Here's how the part is built. I have some questions about the finished solid (model axes, mm). Round coordinates to 2 decimals unless told otherwise and drop trailing zeros. Order: outer loops, then holes, each group sorted by start corner. A loop starts at its lowest first (then second) coordinate and runs counter-clockwise, first axis right, second up. Notation, with made-up numbers: (30.25, 79) -> (37.25, 79) arc R23 ccw to (37.25, 95) -> close; hole circle Ø4 at (26, 75.5). An arc over 180 degrees is marked (long way). Answer in a Markdown table with one row per item.
Autodesk Inventor part; units mm, degrees
ref_plane "YZ Plane" through (0, 0, 0) normal (1, 0, 0) x (0, 1, 0)
ref_plane "XZ Plane" through (0, 0, 0) normal (0, 1, 0) x (-1, 0, 0)
ref_plane "XY Plane" through (0, 0, 0) normal (0, 0, 1) x (1, 0, 0)
sketch "Sketch1" plane through (0, 0, 0) normal (1, 0, 0) x (0, 1, 0)
  line L0 (0, 0) -> (22, 0)
  line L1 (22, 0) -> (22, -31)
  line L2 (22, -31) -> (0, -31)
  line L3 (0, -31) -> (0, 0)
  dimension "d0" = 22
  dimension "d1" = 31
extrude "Extrusion1" add sketch "Sketch1" along normal blind 60
sketch "Sketch2" plane through (60, 0, 0) normal (1, 0, 0) x (0, 0, -1)
  circle A0 centre (1.75, 9.25) radius 1.75
  circle A1 centre (1.75, 12.75) radius 1.75
  line L0 (1.75, 9.25) -> (1.75, 12.75) construction
  line L1 (0, 22) -> (0, 0)
  point P0 (1.75, 11)
  point P1 (0, 11)
  point P2 (1.75, 11)
  dimension "d4" = 3.5
extrude "Extrusion2" add sketch "Sketch2" along normal blind 10 contours A0 | A1
fillet "Fillet1" radius 6.7625 4 edges at (30, 0, 0) (30, 22, 0) (30, 0, -31) (30, 22, -31)
properties part number "Battery"
1. Suppose I cut it at D-D on z = -6. Write out the boundary of the cut face in (x, y).
Numbers:
| item | result |
|---|---|
| outline | (0, 0.04) -> (60, 0.04) -> (60, 21.96) -> (0, 21.96) -> close |
2. Suppose I cut it at A-A on x = 14. Write out the boundary of the cut face in (y, z) (1 decimal), then the cut area to 3 significant figures.
Numbers:
| item | result |
|---|---|
| outline | (0, -24.2) arc R6.8 ccw to (6.8, -31) -> (15.2, -31) arc R6.8 ccw to (22, -24.2) -> (22, -6.8) arc R6.8 ccw to (15.2, 0) -> (6.8, 0) arc R6.8 ccw to (0, -6.8) -> close |
| area | 643 mm2 |
3. Suppose I cut it at C-C on z = -17.5. Write out the boundary of the cut face in (x, y).
Numbers:
| item | result |
|---|---|
| outline | (0, 0) -> (60, 0) -> (60, 22) -> (0, 22) -> close |
4. For pin 1 Ø1 at (x, y) = (36.5, 9.5) entering from +Z; pin 2 Ø10 at (y, z) = (5.5, -18.5) entering from +X; pin 3 Ø1 at (x, z) = (44, -6) entering from -Y; pin 4 Ø3 at (x, y) = (25, 5) entering from -Z, each with a flat end and sliding along its axis, tell me the tip position at first contact or that it passes through.
Numbers:
| item | result |
|---|---|
| pin 1 | stops at z = 0 |
| pin 2 | stops at x = 60 |
| pin 3 | stops at y = 0.01 |
| pin 4 | stops at z = -30.99 |
5. Suppose I cut it at B-B on y = 10. Write out the boundary of the cut face in (x, z).
Numbers:
| item | result |
|---|---|
| outline | (0, -31) -> (60, -31) -> (60, -3.33) -> (70, -3.33) -> (70, -0.17) -> (60, -0.17) -> (60, 0) -> (0, 0) -> close |
6. We'd pull the mould along Y, two halves only. Please class faces 1 (the face through (30, 22, -15)), 2 (the face through (60, 11, -0.4)), 3 (the face through (30, 11, -31)): released by +Y, released by -Y, zero draft, split by the parting line, or undercut.
Numbers:
| item | result |
|---|---|
| face 1 | released by +Y |
| face 2 | undercut |
| face 3 | zero draft |
7. Please list where these lines run through material, in increasing order: line 1 along X through (y, z) = (1, -18); line 2 along Z through (x, y) = (4, 6.5); line 3 along Z through (x, y) = (57.5, 17.75).
Numbers:
| item | result |
|---|---|
| line 1 | x = 0 to 60 |
| line 2 | z = -30.99 to -0.01 |
| line 3 | z = -30.52 to -0.48 |
